Source: CAD feature listing. Evaluate the final solid. Frame: model axes, mm. A direction names the side the tool comes from. Give positions to 0.01 mm unless a question says otherwise; leave off trailing zeros. Write each loop counter-clockwise with the first axis right and the second up, starting at its lowest first coordinate (ties: lowest second). Pieces come first, ordered by that corner, then holes.
```python
from build123d import *

# Parameters (mm, degrees)
ESQUISSE1_W             = 46
ESQUISSE1_H             = 46
ESQUISSE1_W_2           = 40
ESQUISSE1_H_2           = 40
BOSS_EXTRU_1_DEPTH      = 50
ESQUISSE2_W             = 50
ESQUISSE2_H             = 48
ESQUISSE2_W_2           = 42
ESQUISSE2_H_2           = 42
BOSS_EXTRU_2_DEPTH      = 46
ESQUISSE4_W             = 6
ESQUISSE4_H             = 18
ENL_V_MAT_EXTRU_1_DEPTH = 6
ESQUISSE5_R             = 32.5
ESQUISSE5_W             = 42
ESQUISSE5_H             = 42
BOSS_EXTRU_3_DEPTH      = 17
ESQUISSE6_R             = 32.5
ESQUISSE6_R_2           = 2
ESQUISSE6_R_3           = 13
BOSS_EXTRU_4_DEPTH      = 3
CHANFREIN1_SIZE         = 37.637040876
CHANFREIN1_SIZE_2       = 8
BOSS_EXTRU_5_START      = -5
ESQUISSE7_R             = 35
ESQUISSE7_R_2           = 32.5
BOSS_EXTRU_5_DEPTH      = 3.5
CHANFREIN2_SIZE         = 3
ESQUISSE8_R             = 1.5
ENL_V_MAT_EXTRU_2_DEPTH = 136.499077488
ESQUISSE9_R             = 1.5
ENL_V_MAT_EXTRU_3_DEPTH = 13.5


with BuildPart() as part:
    # Esquisse1 → Boss.-Extru.1 (new body)
    with BuildSketch(Plane.XY):
        with Locations((-23, 23)):
            Rectangle(ESQUISSE1_W, ESQUISSE1_H)
        with Locations((-23, 23)):
            Rectangle(ESQUISSE1_W_2, ESQUISSE1_H_2, mode=Mode.SUBTRACT)
    extrude(amount=BOSS_EXTRU_1_DEPTH)

    # Esquisse2 → Boss.-Extru.2 (add)
    with BuildSketch(Plane(origin=(0, 0, 0), x_dir=(0, 0, -1), z_dir=(1, 0, 0))):
        with Locations((-25, 67)):
            Rectangle(ESQUISSE2_W, ESQUISSE2_H)
        with Locations((-25, 67)):
            Rectangle(ESQUISSE2_W_2, ESQUISSE2_H_2, mode=Mode.SUBTRACT)
    extrude(amount=-BOSS_EXTRU_2_DEPTH)

    # Esquisse4 → Enlèv. mat.-Extru.1 (cut)
    with BuildSketch(Plane.XY.offset(50)):
        with Locations((-43, 67)):
            Rectangle(ESQUISSE4_W, ESQUISSE4_H)
    extrude(amount=-ENL_V_MAT_EXTRU_1_DEPTH, mode=Mode.SUBTRACT)

    # Esquisse5 → Boss.-Extru.3 (add)
    with BuildSketch(Plane(origin=(0, 0, 0), x_dir=(0, 0, -1), z_dir=(1, 0, 0))):
        with Locations(Location((-25, 67, 0), (0, 0, 219.715137232))):
            Circle(ESQUISSE5_R)
        with Locations((-25, 67)):
            Rectangle(ESQUISSE5_W, ESQUISSE5_H, mode=Mode.SUBTRACT)
    extrude(amount=BOSS_EXTRU_3_DEPTH)

    # Esquisse6 → Boss.-Extru.4 (add)
    with BuildSketch(Plane(origin=(17, 0, 0), x_dir=(0, 0, -1), z_dir=(1, 0, 0))):
        with Locations(Location((-25, 67, 0), (0, 0, 219.715137232))):
            Circle(ESQUISSE6_R)
        with Locations(Location((-25, 84.5, 0), (0, 0, 90))):
            Circle(ESQUISSE6_R_2, mode=Mode.SUBTRACT)
        with Locations(Location((-7.5, 67, 0), (0, 0, 90))):
            Circle(ESQUISSE6_R_2, mode=Mode.SUBTRACT)
        with Locations(Location((-25, 49.5, 0), (0, 0, 90))):
            Circle(ESQUISSE6_R_2, mode=Mode.SUBTRACT)
        with Locations(Location((-42.5, 67, 0), (0, 0, 90))):
            Circle(ESQUISSE6_R_2, mode=Mode.SUBTRACT)
        with Locations(Location((-25, 67, 0), (0, 0, 90))):
            Circle(ESQUISSE6_R_3, mode=Mode.SUBTRACT)
    extrude(amount=BOSS_EXTRU_4_DEPTH)

    # Chanfrein1
    # the kernel refuses this chamfer: 37.637040876, 8 mm, written as the material it adds along each edge
    with BuildSketch(Plane(origin=(0, 185.543751295, 50), x_dir=(-0.999967974892076, 0, -0.008003073799517018), z_dir=(0, -1, 0))) as chanfrein1_piece_1_section:
        Polygon((CHANFREIN1_SIZE * 0.999967974888, -CHANFREIN1_SIZE * 0.00800307379948), (-CHANFREIN1_SIZE_2 * 0.00800307379952, -CHANFREIN1_SIZE_2 * 0.999967974892), (0, 0), align=None)
    chanfrein1_piece_1 = extrude(amount=237.08750259, mode=Mode.PRIVATE)
    chanfrein1_piece_1 = chanfrein1_piece_1 & Plane(origin=(-15.292244733, 67, 25), x_dir=(0, -0.6389710663806465, 0.7692307692288313), z_dir=(-1, 0, 0)) * Cylinder(32.5, 625, mode=Mode.PRIVATE)
    add(chanfrein1_piece_1)
    with BuildSketch(Plane(origin=(0, 185.543751295, 0), x_dir=(-0.999967974892076, 0, 0.008003073799517044), z_dir=(0, -1, 0))) as chanfrein1_piece_2_section:
        Polygon((CHANFREIN1_SIZE * 0.999967974888, CHANFREIN1_SIZE * 0.00800307379948), (-CHANFREIN1_SIZE_2 * 0.00800307379952, CHANFREIN1_SIZE_2 * 0.999967974892), (0, 0), align=None)
    chanfrein1_piece_2 = extrude(amount=237.08750259, mode=Mode.PRIVATE)
    chanfrein1_piece_2 = chanfrein1_piece_2 & Plane(origin=(-15.292244734, 67, 25), x_dir=(0, -0.6389710663806465, 0.7692307692288313), z_dir=(-1, 0, 0)) * Cylinder(32.5, 625, mode=Mode.PRIVATE)
    add(chanfrein1_piece_2)

    # Esquisse7 → Boss.-Extru.5 (add)
    with BuildSketch(Plane.ZY.offset(BOSS_EXTRU_5_START)):
        with Locations(Location((25, 67, 0), (0, 0, 270))):
            Circle(ESQUISSE7_R)
        with Locations(Location((25, 67, 0), (0, 0, 270))):
            Circle(ESQUISSE7_R_2, mode=Mode.SUBTRACT)
    extrude(amount=-BOSS_EXTRU_5_DEPTH)

    # Chanfrein2
    # the kernel refuses this chamfer: 3 mm, written as the material it adds along each edge
    with BuildSketch(Plane(origin=(5, 67, 25), x_dir=(0, -0.6389710663806288, 0.7692307692288458), z_dir=(0, -0.7692307692288458, -0.6389710663806288))) as chanfrein2_piece_1_section:
        Polygon((32.5 + CHANFREIN2_SIZE, 0), (32.5, CHANFREIN2_SIZE), (32.5, 0), align=None)
    chanfrein2_piece_1 = revolve(axis=Axis((5, 67, 25), (-1, 0, 0)), mode=Mode.PRIVATE)
    chanfrein2_piece_1 = chanfrein2_piece_1 & Plane(origin=(3.278266852, 67, 25), x_dir=(0, -1, 0), z_dir=(-1, 0, 0)) * Cylinder(35, 142, mode=Mode.PRIVATE)
    add(chanfrein2_piece_1)

    # Esquisse8 → Enlèv. mat.-Extru.2 (cut, through all)
    with BuildSketch(Plane.ZY.offset(46)):
        with Locations(Location((25, 23, 0), (0, 0, 270))):
            Circle(ESQUISSE8_R)
    extrude(amount=-ENL_V_MAT_EXTRU_2_DEPTH, mode=Mode.SUBTRACT)

    # Esquisse9 → Enlèv. mat.-Extru.3 (cut)
    with BuildSketch(Plane.XZ):
        with Locations(Location((-23, 25, 0), (0, 0, 270))):
            Circle(ESQUISSE9_R)
    extrude(amount=-ENL_V_MAT_EXTRU_3_DEPTH, mode=Mode.SUBTRACT)


solid = part.part
```
1. Mould query, pull axis Z, two halves, no side actions, for faces 4 (the cylindrical face through (-8.365, 46.352, -0.098)), 5 (the flat face through (-15, 88, 25)), 6 (the flat face through (-43, 58, 48)). Classes: +Z half, -Z half, draft (parallel to the pull), parting line (faces both ways), or undercut.
2. Cut plane B-B, the plane y = 67. State how many separate pieces and enclosed holes the cut face has, then the cut area to 3 significant figures.
3. Cut plane D-D, the plane x = 13. Return the cut outline in (y, z), then the cut area to 3 significant figures.
4. Cut plane A-A, the plane x = -16.5. Return the cut outline in (y, z).
5. Line query: L1, parallel to Y at x = -13, z = 8; L2, parallel to Z at x = 17.7, y = 67; L3, parallel to X at y = 10, z = 5. Output: solid intervals per line, ascending.
6. Cut plane C-C, the plane x = -41.5. Return the cut outline in (y, z), then the cut area to 3 significant figures.
7. Contact query for flat-ended pins moving along their axis: P1, Ø1.5, axis at y = 13.5, z = 23.5, coming from the +X side; P2, Ø8, axis at x = -29, y = 62, coming from the +Z side; P3, Ø6, axis at x = -31.5, y = 82, coming from the -Z side; P4, Ø1.8, axis at y = 23, z = 25, coming from the +X side. Output: stop coordinate, or through.
8. Access query for faces 1 (the flat face through (-23, 91, 25)), 2 (the flat face through (0, 90, 49)), 3 (the cylindrical face through (6.47, 34.67, 11.59)). Directions: +Z, -Z, +X, -X, +Y, -Y. A direction counts if a zero-diameter tool reaches every point of the face in a straight line with its end or side. Return the directions, or none.
Response values:
1. face 4: parting line
1. face 5: undercut
1. face 6: draft
2. separate pieces: 4
2. enclosed holes: 0
2. area: 1,150 mm2
3. outline: circle Ø65 at (67, 25); hole (46, 4) - (88, 4) - (88, 46) - (46, 46) - close
3. area: 1,550 mm2
4. outline: (0, 0) - (3, 0) - (3, 50) - (0, 50) - close; (43, 0) - (46.23, 0) arc R32.5 ccw to (53.35, -4.49) - (80.65, -4.49) arc R32.5 ccw to (87.77, 0) - (91, 0) - (91, 50) - (87.77, 50) arc R32.5 ccw to (80.65, 54.49) - (53.35, 54.49) arc R32.5 ccw to (46.23, 50) - (43, 50) - close; hole (46, 4) - (88, 4) - (88, 46) - (46, 46) - close
5. L1: y = 0 to 3, 43 to 46, 88 to 91
5. L2: z = -7.5 to 5.5, 9.5 to 12, 38 to 40.5, 44.5 to 57.5
5. L3: x = -46 to -43, -3 to 0
6. outline: (0, 0) - (3, 0) - (3, 50) - (0, 50) - close; (43, 0) - (91, 0) - (91, 50) - (76, 50) - (76, 46) - (88, 46) - (88, 4) - (46, 4) - (46, 46) - (58, 46) - (58, 50) - (43, 50) - close
6. area: 714 mm2
7. P1: stops at x = 0
7. P2: stops at z = 52.69
7. P3: stops at z = -1.94
7. P4: passes through
8. face 1: +Z, -Z, -X, +Y
8. face 2: +Z, +Y
8. face 3: +X
